from build123d import *

# Parameters (mm, degrees)
SKETCH_1_W      = 4
SKETCH_1_H      = 10
EXTRUDE_1_DEPTH = 2


with BuildPart() as part:
    # 草图1 → 凸台-拉伸1 (new, symmetric)
    with BuildSketch(Plane.XY):
        Polygon((-46, 0), (-37, 0), (-37, 20), (-46, 20), (-52, 20), (-52, 0), align=None)
        with Locations((-48, 10)):
            Rectangle(SKETCH_1_W, SKETCH_1_H, mode=Mode.SUBTRACT)
        with Locations((-41, 10)):
            Rectangle(SKETCH_1_W, SKETCH_1_H, mode=Mode.SUBTRACT)
    extrude(amount=EXTRUDE_1_DEPTH, both=True)


solid = part.part
Can you work these out from the model? Positions are in its coordinate system, mm. A direction names the side the tool comes from. Coordinates: 2 decimals unless noted, no trailing zeros. Loops run counter-clockwise (first coordinate to the right, second up) from the corner with the lowest first, then second, coordinate; pieces in that order, holes last. Notation, with made-up numbers: (-11.5, 52) - (26.5, 52) arc R38 cw to (26.5, 91) - close; hole circle Ø3 at (12, 7.5). An arc over 180 degrees is marked (long way). Put each result on its own line as item: value. Start each with the question number.
Item 1: Suppose I cut it at B-B (x = -47.75). Please give me the cut outline in (y, z), and give its area (3 significant figures).
Item 2: If I drill on line 1 along X through (y, z) = (6, -0.9); line 2 along Y through (x, z) = (-48.75, 1.1), over which ranges is the centre line in solid material (lowest first)?
Item 3: Suppose I cut it at C-C (y = 7.75). Please give me the cut outline in (x, z).
Item 4: Suppose I cut it at A-A (z = 0.7). Please give me the cut outline in (x, y).
Item 5: Which directions (+Z, -Z, +X, -X, +Y, -Y) give clear straight access to the entire face, cutting with the end or side of a thin tool? Please do faces 1 (the face through (-41, 5, 0)), 2 (the face through (-45, 10, -2)).
Item 6: If we mould it in two halves opening along X, with no side actions, what happens to faces 3 (the face through (-41, 15, 0)), 4 (the face through (-44, 20, 0)), 5 (the face through (-37, 10, 0)), 6 (the face through (-52, 10, 0))? For each: +X half, -X half, draft (parallel to the pull), parting line (faces both ways), or undercut.
Here are the results:
1. outline: (0, -2) - (5, -2) - (5, 2) - (0, 2) - close; (15, -2) - (20, -2) - (20, 2) - (15, 2) - close
1. area: 40.0 mm²
2. line 1: -52 to -50, -46 to -43, -39 to -37
2. line 2: 0 to 5, 15 to 20
3. outline: (-52, -2) - (-50, -2) - (-50, 2) - (-52, 2) - close; (-46, -2) - (-43, -2) - (-43, 2) - (-46, 2) - close; (-39, -2) - (-37, -2) - (-37, 2) - (-39, 2) - close
4. outline: (-52, 0) - (-37, 0) - (-37, 20) - (-52, 20) - close; hole (-50, 5) - (-46, 5) - (-46, 15) - (-50, 15) - close; hole (-43, 5) - (-39, 5) - (-39, 15) - (-43, 15) - close
5. face 1: +Z, -Z
5. face 2: -Z, +X, -X, +Y, -Y
6. face 3: undercut
6. face 4: draft
6. face 5: +X half
6. face 6: -X half
